Design review of the part built by this model. Coordinates are the model's own, in mm. A direction names the side the tool comes from. Round coordinates to 2 decimals unless told otherwise and drop trailing zeros. Write each loop counter-clockwise with the first axis right and the second up, starting at its lowest first coordinate (ties: lowest second). Pieces come first, ordered by that corner, then holes. Notation, with made-up numbers: (2.5, 20.5) -> (29.5, 20.5) arc R33 ccw to (29.5, 54.5) -> close; hole circle Ø10 at (89, 2). An arc over 180 degrees is marked (long way). Write item = value, one per line. Start each with the question number.
Item 1: Machinability: for faces 4 (the flat face through (3, -1, 1)), 5 (the flat face through (9, -5, 75)), 6 (the flat face through (28, -27, 49)), which of the approach directions +Z, -Z, +X, -X, +Y, -Y give a long, thin tool a straight path to every point of the face, cutting with its end or side? Answer none if there is none.
Item 2: Add section A-A, the plane x = 13.75. State the section outline as (y, z) points, then the cut area to 3 significant figures.
Item 3: To check wall thickness, follow L1, parallel to Z at x = 6, y = 0; L2, parallel to X at y = -6, z = -5.5; L3, parallel to Z at x = 14, y = -38.5. State the ranges of each line that lie inside material, in increasing order.
Item 4: Mouldability with a two-part tool opening along Z and no side actions: class faces 1 (the cylindrical face through (4.437, -3.461, -81.654)), 2 (the flat face through (18, -21, 61)), 3 (the cylindrical face through (24.71, -2.64, -59.94)) as released by +Z, released by -Z, zero draft, split by the parting line, or undercut.
Item 5: For pin 1 Ø11.5 at (y, z) = (0, 75) entering from +X; pin 2 Ø1 at (x, y) = (5, -38.5) entering from +Z; pin 3 Ø1.5 at (x, y) = (8, 22.5) entering from -Z, all flat-tipped, find the tip position at first contact; note any pin that passes through.
from build123d import *

# Parameters (mm, degrees)
F3_D           = 9
F3_DEPTH       = 18
F3_CBORE_D     = 15
F3_CBORE_DEPTH = 9
F4_R           = 4
F5_SIZE        = 0.5
F6_R           = 4
F7_SIZE        = 1


with BuildPart() as f1:
    # F0 (on Front) → F1 (revolve)
    with BuildSketch(Plane.XZ):
        Polygon((18, 90), (0, 90), (0, 0), (3, 0), (3, 55), (28, 55), (28, 60), (18, 60), align=None)
    revolve(axis=Axis((1.5, 0, 0), (1, 0, 0)))

    # F3
    with Locations(Plane(origin=(0, 0, 0), x_dir=(0, -1, 0), z_dir=(-1, 0, 0))):
        with Locations((0, 75), (75, 0), (0, -75), (-75, 0)):
            CounterBoreHole(F3_D / 2, F3_CBORE_D / 2, F3_CBORE_DEPTH, depth=F3_DEPTH)

    # F4
    f4_edges = [f1.edges().sort_by_distance(p)[0] for p in [
        (18, 0, -60),
    ]]
    fillet(f4_edges, radius=F4_R)

    # F5
    f5_edges = [f1.edges().sort_by_distance(p)[0] for p in [
        (28, 0, -60),
        (28, 0, -55),
    ]]
    chamfer(f5_edges, length=F5_SIZE)

    # F6
    f6_edges = [f1.edges().sort_by_distance(p)[0] for p in [
        (3, 0, -55),
    ]]
    fillet(f6_edges, radius=F6_R)

    # F7
    f7_edges = [f1.edges().sort_by_distance(p)[0] for p in [
        (0, 0, -90),
    ]]
    chamfer(f7_edges, length=F7_SIZE)


solid = f1.part
Result set:
q1.face_4 = +X
q1.face_5 = -X
q1.face_6 = +Z, -Z, +X, +Y, -Y
q2.outline = circle Ø180 at (0, 0); hole circle Ø9 at (-75, 0); hole circle Ø110 at (0, 0); hole circle Ø9 at (0, -75); hole circle Ø9 at (0, 75); hole circle Ø9 at (75, 0)
q2.area = 15,700 mm²
q3.L1 = -90 to -82.5, -67.5 to -54.87, 54.87 to 67.5, 82.5 to 90
q3.L2 = 0 to 3
q3.L3 = -81.35 to -39.28, 39.28 to 81.35
q4.face_1 = undercut
q4.face_2 = zero draft
q4.face_3 = split by the parting line
q5.pin_1 = 18
q5.pin_2 = 81.58
q5.pin_3 = -87.33
